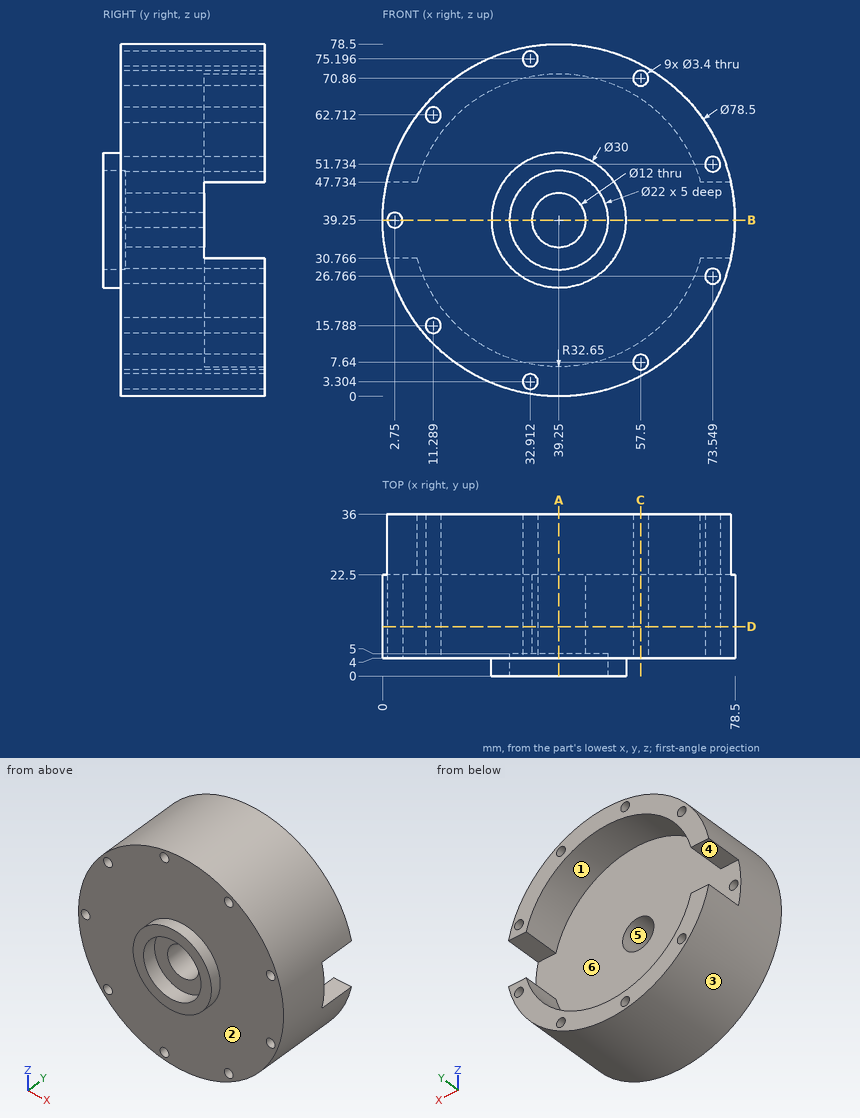
Job drawing, mm, ordinate dimensions from the low corner. One solid piece. A direction names the side the tool comes from. Coordinates: 2 decimals unless noted, no trailing zeros. Order: outer loops, then holes, each group sorted by start corner. A loop starts at its lowest first (then second) coordinate and runs counter-clockwise, first axis right, second up. Notation, with made-up numbers: (47, 18.25) - (106, 18.25) arc R37 ccw to (106, 56.25) - close; hole circle Ø3 at (53.5, 33). An arc over 180 degrees is marked (long way). Write each question's results on one line, items separated by ' | '. Start each with the question number.
Item 1: Band-saw the part on C-C on x = 57.5. Write the cut outline in (y, z), and give its area (3 significant figures).
Item 2: Band-saw the part on D-D on y = 11. State how many separate pieces and enclosed holes the cut face has, and give its area (4 significant figures).
Item 3: Flat gauge pins, fed straight in: pin 1 (7.5 mm diameter, centred on x = 6, y = 26.5, fed in from -Z); pin 2 (4 mm diameter, centred on x = 11.29, z = 15.79, fed in from -Y); pin 3 (13 mm diameter, centred on x = 39.25, z = 39.25, fed in from -Y). Where does each tip first touch, or does it go through?
Item 4: Wall check: probe 1 along X at (y, z) = (29, 27.5) (1 decimal); probe 2 along Z at (x, y) = (39.25, 2.85); probe 3 along Z at (x, y) = (39, 18) (1 decimal). Give the ranges that are in metal, low to high. Write a range as [from, to].
Item 5: Band-saw the part on A-A on x = 39.25. Write the cut outline in (y, z), and give its area (3 significant figures).
Item 6: Tool access for the marked faces 4, 5 and 6: list every direction of +Z, -Z, +X, -X, +Y, -Y with a clear straight run to the whole face (end or side of a thin tool).
Item 7: Band-saw the part on B-B on z = 39.25. Write the cut outline in (x, y).
Item 8: Mould opens along Z. For the marked faces 1, 2 and 3 say: released by +Z, released by -Z, zero draft, split by the parting line, or undercut.
Numbers:
1) outline: (4, 4.5) - (36, 4.5) - (36, 5.94) - (4, 5.94) - close; (4, 9.34) - (36, 9.34) - (36, 12.18) - (22.5, 12.18) - (22.5, 66.32) - (36, 66.32) - (36, 69.16) - (4, 69.16) - close; (4, 72.56) - (36, 72.56) - (36, 74) - (4, 74) - close | area: 1,280 mm^2
2) separate pieces: 1 | enclosed holes: 10 | area: 4,645 mm^2
3) pin 1: z = 13.36 | pin 2: y = 4 | pin 3: y = 5
4) probe 1: [1.8, 8.8], [69.7, 72], [75.1, 76.7] | probe 2: [24.25, 28.25], [50.25, 54.25] | probe 3: [0, 33.3], [45.2, 78.5]
5) outline: (0, 24.25) - (4, 24.25) - (4, 0) - (36, 0) - (36, 6.6) - (22.5, 6.6) - (22.5, 33.25) - (5, 33.25) - (5, 28.25) - (0, 28.25) - close; (0, 50.25) - (5, 50.25) - (5, 45.25) - (22.5, 45.25) - (22.5, 71.9) - (36, 71.9) - (36, 78.5) - (4, 78.5) - (4, 54.25) - (0, 54.25) - close | area: 1,430 mm^2
6) face 4: +X, -X, +Y | face 5: +Y, -Y | face 6: +Y
7) outline: (0, 4) - (1.05, 4) - (1.05, 22.5) - (0, 22.5) - close; (4.45, 4) - (24.25, 4) - (24.25, 0) - (28.25, 0) - (28.25, 5) - (33.25, 5) - (33.25, 22.5) - (4.45, 22.5) - close; (45.25, 5) - (50.25, 5) - (50.25, 0) - (54.25, 0) - (54.25, 4) - (78.5, 4) - (78.5, 22.5) - (45.25, 22.5) - close
8) face 1: undercut | face 2: zero draft | face 3: split by the parting line
